```python
from build123d import *

# Parameters (mm, degrees)
IZIM1_W                     = 40
IZIM1_H                     = 20
Y_KSEKLIK_EKSTR_ZYON1_DEPTH = 30
IZIM2_W                     = 55
IZIM2_H                     = 20
Y_KSEKLIK_EKSTR_ZYON2_DEPTH = 3
IZIM3_R                     = 2.647008292
KES_EKSTR_ZYON1_DEPTH       = 13
IZIM4_R                     = 10.060368761
Y_KSEKLIK_EKSTR_ZYON3_DEPTH = 3
IZIM5_R                     = 7.317651021
Y_KSEKLIK_EKSTR_ZYON4_DEPTH = 2
IZIM6_R                     = 3.5
Y_KSEKLIK_EKSTR_ZYON5_DEPTH = 10


with BuildPart() as part:
    # Çizim1 → Yükseklik-Ekstrüzyon1 (new body)
    with BuildSketch(Plane(origin=(0, 0, 0), x_dir=(1, 0, 0), z_dir=(0, 1, 0))):
        Rectangle(IZIM1_W, IZIM1_H)
    extrude(amount=Y_KSEKLIK_EKSTR_ZYON1_DEPTH)

    # Çizim2 → Yükseklik-Ekstrüzyon2 (add)
    with BuildSketch(Plane(origin=(0, 22, 0), x_dir=(1, 0, 0), z_dir=(0, 1, 0))):
        Rectangle(IZIM2_W, IZIM2_H)
    extrude(amount=Y_KSEKLIK_EKSTR_ZYON2_DEPTH)

    # Çizim3 → Kes-Ekstrüzyon1 (cut)
    with BuildSketch(Plane(origin=(0, 25, 0), x_dir=(1, 0, 0), z_dir=(0, 1, 0))):
        with Locations(Location((-23.75, 5.00174063, 0), (0, 0, 270))):
            Circle(IZIM3_R)
        with Locations(Location((-23.75, -5.00174063, 0), (0, 0, 90))):
            Circle(IZIM3_R)
        with Locations(Location((23.75, -5.00174063, 0), (0, 0, 270))):
            Circle(IZIM3_R)
        with Locations(Location((23.75, 5.00174063, 0), (0, 0, 90))):
            Circle(IZIM3_R)
    extrude(amount=-KES_EKSTR_ZYON1_DEPTH, mode=Mode.SUBTRACT)

    # Çizim4 → Yükseklik-Ekstrüzyon3 (add)
    with BuildSketch(Plane(origin=(0, 30, 0), x_dir=(1, 0, 0), z_dir=(0, 1, 0))):
        with Locations(Location((-9.631551276, 0, 0), (0, 0, 96.279921615))):
            Circle(IZIM4_R)
    extrude(amount=Y_KSEKLIK_EKSTR_ZYON3_DEPTH)

    # Çizim5 → Yükseklik-Ekstrüzyon4 (add)
    with BuildSketch(Plane(origin=(0, 33, 0), x_dir=(1, 0, 0), z_dir=(0, 1, 0))):
        with Locations(Location((-9.631551276, 0, 0), (0, 0, 270))):
            Circle(IZIM5_R)
    extrude(amount=Y_KSEKLIK_EKSTR_ZYON4_DEPTH)

    # Çizim6 → Yükseklik-Ekstrüzyon5 (add)
    with BuildSketch(Plane(origin=(0, 35, 0), x_dir=(1, 0, 0), z_dir=(0, 1, 0))):
        with Locations(Location((-9.631551276, 0, 0), (0, 0, 270))):
            Circle(IZIM6_R)
    extrude(amount=Y_KSEKLIK_EKSTR_ZYON5_DEPTH)


solid = part.part
```
For this review, take the finished solid that the model builds, in its own axes (mm). A direction names the side the tool comes from. Round coordinates to 2 decimals unless told otherwise and drop trailing zeros. Order: outer loops, then holes, each group sorted by start corner. A loop starts at its lowest first (then second) coordinate and runs counter-clockwise, first axis right, second up. Notation, with made-up numbers: (21, 61) -> (60, 61) arc R9 ccw to (60, 69) -> close; hole circle Ø5 at (14.25, 86). An arc over 180 degrees is marked (long way). Use a Markdown table: item, result.
Item 1: Take a section at D-D (y = 13.5). State the section outline as (x, z) points.
Resolved:
| item | result |
|---|---|
| outline | (-20, -10) -> (20, -10) -> (20, 10) -> (-20, 10) -> close |
Item 2: Take a section at B-B (z = 0). State the section outline as (x, y) points, plus the area to 3 significant figures.
Resolved:
| item | result |
|---|---|
| outline | (-27.5, 22) -> (-20, 22) -> (-20, 0) -> (20, 0) -> (20, 22) -> (27.5, 22) -> (27.5, 25) -> (20, 25) -> (20, 30) -> (0.43, 30) -> (0.43, 33) -> (-2.31, 33) -> (-2.31, 35) -> (-6.13, 35) -> (-6.13, 45) -> (-13.13, 45) -> (-13.13, 35) -> (-16.95, 35) -> (-16.95, 33) -> (-19.69, 33) -> (-19.69, 30) -> (-20, 30) -> (-20, 25) -> (-27.5, 25) -> close |
| area | 1,400 mm² |
Item 3: For line 1 along X through (y, z) = (23.5, -3); line 2 along X through (y, z) = (19.5, -1.25); line 3 along Y through (x, z) = (3, -8.25), list the stretches that pass through material, from the lowest coordinate up. Write a range as [from, to].
Resolved:
| item | result |
|---|---|
| line 1 | x = [-27.5, -25.48], [-22.02, 22.02], [25.48, 27.5] |
| line 2 | x = [-20, 20] |
| line 3 | y = [0, 30] |
Item 4: For pin 1 (6 mm diameter, centred on x = 22.5, z = -0.5, fed in from +Y); pin 2 (10 mm diameter, centred on y = 13.5, z = -8, fed in from +X); pin 3 (5 mm diameter, centred on x = -23.75, z = -5, fed in from -Y); pin 4 (2 mm diameter, centred on x = -24, z = -0.5, fed in from +Y), all flat-tipped, find the tip position at first contact; note any pin that passes through.
Resolved:
| item | result |
|---|---|
| pin 1 | stops at y = 30 |
| pin 2 | stops at x = 20 |
| pin 3 | passes through |
| pin 4 | stops at y = 25 |
Item 5: Machinability: for faces 1 (the flat face through (24, 25, 0)), 2 (the flat face through (-24, 22, 0)), 3 (the cylindrical face through (-6.16, 39.93, -0.46)), 4 (the flat face through (24, 22, 0)), which of the approach directions +Z, -Z, +X, -X, +Y, -Y give a long, thin tool a straight path to every point of the face, cutting with its end or side? Answer none if there is none.
Resolved:
| item | result |
|---|---|
| face 1 | +Z, -Z, +X, +Y |
| face 2 | +Z, -Z, -X, -Y |
| face 3 | +Y |
| face 4 | +Z, -Z, +X, -Y |
Item 6: Draft analysis for pull direction X (two halves, no side actions). For faces 5 (the cylindrical face through (-26.374, 23.521, 5.346)), 6 (the cylindrical face through (-2.376, 33.986, -0.953)), 7 (the flat face through (-2, 33, -2)), state which applies: +X half, -X half, draft (parallel to the pull), parting line (faces both ways), or undercut.
Resolved:
| item | result |
|---|---|
| face 5 | undercut |
| face 6 | parting line |
| face 7 | draft |
Item 7: Take a section at A-A (x = 23.75). State the section outline as (y, z) points.
Resolved:
| item | result |
|---|---|
| outline | (22, -10) -> (25, -10) -> (25, -7.65) -> (22, -7.65) -> close; (22, -2.35) -> (25, -2.35) -> (25, 2.35) -> (22, 2.35) -> close; (22, 7.65) -> (25, 7.65) -> (25, 10) -> (22, 10) -> close |
Item 8: Take a section at C-C (z = -5.25). State the section outline as (x, y) points, plus the area to 3 significant figures.
Resolved:
| item | result |
|---|---|
| outline | (-27.5, 22) -> (-26.39, 22) -> (-26.39, 25) -> (-27.5, 25) -> close; (-21.11, 22) -> (-20, 22) -> (-20, 0) -> (20, 0) -> (20, 22) -> (21.11, 22) -> (21.11, 25) -> (20, 25) -> (20, 30) -> (-1.05, 30) -> (-1.05, 33) -> (-4.53, 33) -> (-4.53, 35) -> (-14.73, 35) -> (-14.73, 33) -> (-18.21, 33) -> (-18.21, 30) -> (-20, 30) -> (-20, 25) -> (-21.11, 25) -> close; (26.39, 22) -> (27.5, 22) -> (27.5, 25) -> (26.39, 25) -> close |
| area | 1,290 mm² |
